Geometry check sheet. Reference: the model listing, model coordinates, mm. Give positions to 0.01 mm unless a question says otherwise; leave off trailing zeros. Loops run counter-clockwise (first coordinate to the right, second up) from the corner with the lowest first, then second, coordinate; pieces in that order, holes last. Notation, with made-up numbers: (89.25, 2.5) -> (125.25, 2.5) arc R10 ccw to (125.25, 19.5) -> close; hole circle Ø10 at (-30.75, 14). An arc over 180 degrees is marked (long way). Write each question's results on one line, items separated by ' | '. Start each with the question number.
1) Depth check by flat-ended pin: pin 1 (1 mm diameter, centred on x = 19.5, z = 1, fed in from +Y); pin 2 (0.6 mm diameter, centred on x = 60, z = 1, fed in from +Y); pin 3 (1 mm diameter, centred on y = 17.5, z = 0.5, fed in from -X). Enter the tip coordinate at first touch or a pass-through.
2) Sectioned sample at D-D on x = 54. Record the cut outline in (y, z).
3) Sectioned sample at B-B on y = 6.5. Record the cut outline in (x, z).
4) Sectioned sample at A-A on y = 18.75. Record the cut outline in (x, z), then the cut area to 3 significant figures.
5) Scan lines: line 1 (X direction, y = 12.5, z = 1.55); line 2 (X direction, y = 7.5, z = 0.2); line 3 (X direction, y = 16.75, z = 0.6). Record each from-to range of solid material in increasing order. Write a range as from..to.
6) Sectioned sample at C-C on z = 1.6. Record the cut outline in (x, y).
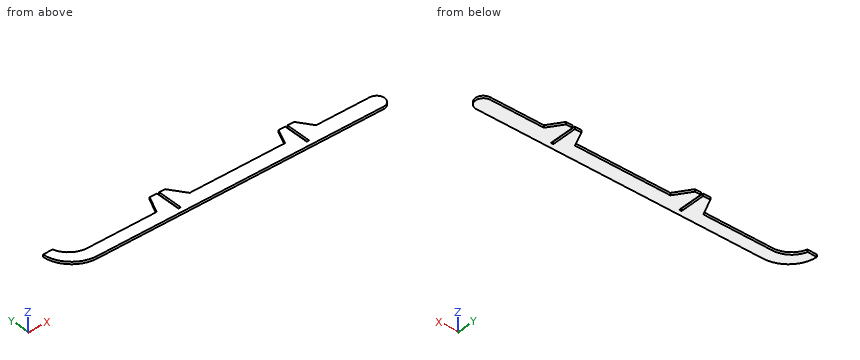
```python
from build123d import *

# Parameters (mm, degrees)
RESSALTO_EXTRUS_O1_DEPTH = 2


with BuildPart() as part:
    # Esboço1 → Ressalto-extrusão1 (new body)
    with BuildSketch(Plane.XY):
        with BuildLine():
            Line((78.907701248, 0), (-161.092298752, 0))
            ThreePointArc((-161.092298752, 0), (-178.278212695, 6.861020331), (-186.013965864, 23.671355275))
            Line((-186.013965864, 23.671355275), (-178.013965864, 23.671355275))
            ThreePointArc((-178.013965864, 23.671355275), (-171.273030794, 14.060352601), (-160.128605048, 10.370724866))
            Line((-160.128605048, 10.370724866), (-102.128605048, 10.370724866))
            Line((-102.128605048, 10.370724866), (-95.535452379, 25))
            Line((-95.535452379, 25), (-89.442008497, 25))
            Line((-89.442008497, 25), (-89.442008497, 4))
            Line((-89.442008497, 4), (-87.442008497, 4))
            Line((-87.442008497, 4), (-87.442008497, 25))
            Line((-87.442008497, 25), (-82.535452379, 25))
            Line((-82.535452379, 25), (-73.291416334, 11.883859156))
            Line((-73.291416334, 11.883859156), (6.708583666, 11.883859156))
            Line((6.708583666, 11.883859156), (12.619793773, 25))
            Line((12.619793773, 25), (18.119793773, 25))
            Line((18.119793773, 25), (18.119793773, 4))
            Line((18.119793773, 4), (20.119793773, 4))
            Line((20.119793773, 4), (20.119793773, 25))
            Line((20.119793773, 25), (25.619793773, 25))
            Line((25.619793773, 25), (33.907701248, 13.240487032))
            Line((33.907701248, 13.240487032), (78.907701248, 13.240487032))
            ThreePointArc((78.907701248, 13.240487032), (85.527944764, 6.620243516), (78.907701248, 0))
        make_face()
    extrude(amount=RESSALTO_EXTRUS_O1_DEPTH)


solid = part.part
```
Result:
1) pin 1: y = 4 | pin 2: y = 13.24 | pin 3: x = -185.06
2) outline: (0, 0) -> (13.24, 0) -> (13.24, 2) -> (0, 2) -> close
3) outline: (-177.89, 0) -> (-89.44, 0) -> (-89.44, 2) -> (-177.89, 2) -> close; (-87.44, 0) -> (18.12, 0) -> (18.12, 2) -> (-87.44, 2) -> close; (20.12, 0) -> (85.53, 0) -> (85.53, 2) -> (20.12, 2) -> close
4) outline: (-185.26, 0) -> (-175.71, 0) -> (-175.71, 2) -> (-185.26, 2) -> close; (-98.35, 0) -> (-89.44, 0) -> (-89.44, 2) -> (-98.35, 2) -> close; (-87.44, 0) -> (-78.13, 0) -> (-78.13, 2) -> (-87.44, 2) -> close; (9.8, 0) -> (18.12, 0) -> (18.12, 2) -> (9.8, 2) -> close; (20.12, 0) -> (30.02, 0) -> (30.02, 2) -> (20.12, 2) -> close | area: 92.0 mm^2
5) line 1: -182.72..-168.79, -101.17..-89.44, -87.44..-73.73, 6.99..18.12, 20.12..81.95 | line 2: -178.93..-89.44, -87.44..18.12, 20.12..85.47 | line 3: -184.66..-174.18, -99.25..-89.44, -87.44..-76.72, 8.9..18.12, 20.12..31.43
6) outline: (-186.01, 23.67) arc R24.95 ccw to (-161.09, 0) -> (78.91, 0) arc R6.62 ccw to (78.91, 13.24) -> (33.91, 13.24) -> (25.62, 25) -> (20.12, 25) -> (20.12, 4) -> (18.12, 4) -> (18.12, 25) -> (12.62, 25) -> (6.71, 11.88) -> (-73.29, 11.88) -> (-82.54, 25) -> (-87.44, 25) -> (-87.44, 4) -> (-89.44, 4) -> (-89.44, 25) -> (-95.54, 25) -> (-102.13, 10.37) -> (-160.13, 10.37) arc R18.68 cw to (-178.01, 23.67) -> close
